Source: CAD feature listing. Evaluate the final solid. Frame: model axes, mm. A direction names the side the tool comes from. Round coordinates to 2 decimals unless told otherwise and drop trailing zeros. Write each loop counter-clockwise with the first axis right and the second up, starting at its lowest first coordinate (ties: lowest second). Pieces come first, ordered by that corner, then holes. Notation, with made-up numbers: M 47.5,-22.5 L 100.5,-22.5 A31 ccw 100.5,6.5 Z; hole C 82.5,68 d9. An arc over 180 degrees is marked long. Use a Markdown table: item, result.
```python
from build123d import *

# Parameters (mm, degrees)
SKETCH1_R           = 12
SKETCH1_R_2         = 5.5
BOSS_EXTRUDE1_DEPTH = 3
SKETCH1_5_R         = 5.5
SKETCH1_5_R_2       = 3
BOSS_EXTRUDE3_DEPTH = 12
FILLET2_R           = 2
CUT_EXTRUDE1_START  = -5.5
SKETCH2_R           = 1.6
CUT_EXTRUDE1_DEPTH  = 11
SKETCH3_R           = 2.001151749
CUT_EXTRUDE2_DEPTH  = 4


with BuildPart() as part:
    # Sketch1 → Boss-Extrude1 (new body)
    with BuildSketch(Plane.XY):
        Circle(SKETCH1_R)
        Circle(SKETCH1_R_2, mode=Mode.SUBTRACT)
    extrude(amount=BOSS_EXTRUDE1_DEPTH)

    # Sketch1<5> → Boss-Extrude3 (add)
    with BuildSketch(Plane.XY):
        Circle(SKETCH1_5_R)
        Circle(SKETCH1_5_R_2, mode=Mode.SUBTRACT)
    extrude(amount=BOSS_EXTRUDE3_DEPTH)

    # Fillet2
    fillet2_edges = [part.edges().sort_by_distance(p)[0] for p in [
        (-5.5, 0, 3),
    ]]
    fillet(fillet2_edges, radius=FILLET2_R)

    # Sketch2 → Cut-Extrude1 (cut)
    with BuildSketch(Plane(origin=(0, 0, 0), x_dir=(1, 0, 0), z_dir=(0, 1, 0)).offset(CUT_EXTRUDE1_START)):
        with Locations(Location((0, -7.949486667, 0), (0, 0, 90))):
            Circle(SKETCH2_R)
    extrude(amount=CUT_EXTRUDE1_DEPTH, mode=Mode.SUBTRACT)

    # Sketch3 → Cut-Extrude2 (cut)
    with BuildSketch(Plane.XY.offset(3)):
        with Locations((0, 8.599839423)):
            Circle(SKETCH3_R)
        with Locations((7.447679409, -4.299919712)):
            Circle(SKETCH3_R)
        with Locations((-7.447679409, -4.299919712)):
            Circle(SKETCH3_R)
    extrude(amount=-CUT_EXTRUDE2_DEPTH, mode=Mode.SUBTRACT)


solid = part.part
```
Q1. Reachability of faces 1 (the cylindrical face through (-8.923, -2.947, 1.521)), 2 (the cylindrical face through (5.08, -2.11, 8.45)), 3 (the flat face through (2.4, -2.4, 12)) from +Z, -Z, +X, -X, +Y, -Y: full face, straight path, thin tool, end or side. Return the list, or none.
Results are:
| item | result |
|---|---|
| face 1 | -Z |
| face 2 | +Z |
| face 3 | +Z, +X, -X, +Y, -Y |
Q2. Line query: L1, parallel to Y at x = 0, z = 0.7; L2, parallel to Z at x = 7.75, y = 7; L3, parallel to X at y = 3, z = 6.5. Output: solid intervals per line, ascending.
Results are:
| item | result |
|---|---|
| L1 | -12 to -3, 3 to 6.6, 10.6 to 12 |
| L2 | 0 to 3 |
| L3 | -4.61 to -0.68, 0.68 to 4.61 |
Q3. First-contact query: pin 1 Ø3 at (x, z) = (-6, 1) entering from +Y; pin 2 Ø2.5 at (x, y) = (-7.45, -4.3) entering from -Z; pin 3 Ø3.5 at (x, z) = (0, 7.95) entering from +Y. Flat tips, straight axial feed; report the tip coordinate or a pass-through.
Results are:
| item | result |
|---|---|
| pin 1 | y = 11.12 |
| pin 2 | z = 3 |
| pin 3 | y = 5.5 |
Q4. Section B-B on x = 0. Return loops of the section in (y, z).
Results are:
| item | result |
|---|---|
| outline | M -12,0 L -3,0 L -3,6.35 L -5.5,6.35 L -5.5,5 A2 cw -7.5,3 L -12,3 Z; M -5.5,9.55 L -3,9.55 L -3,12 L -5.5,12 Z; M 3,0 L 6.6,0 L 6.6,3 L 7.5,3 A2 cw 5.5,5 L 5.5,6.35 L 3,6.35 Z; M 3,9.55 L 5.5,9.55 L 5.5,12 L 3,12 Z; M 10.6,0 L 12,0 L 12,3 L 10.6,3 Z |
Q5. Section A-A on y = 0. Return loops of the section in (x, z), plus the area to 3 significant figures.
Results are:
| item | result |
|---|---|
| outline | M -12,0 L -3,0 L -3,12 L -5.5,12 L -5.5,5 A2 cw -7.5,3 L -12,3 Z; M 3,0 L 12,0 L 12,3 L 7.5,3 A2 cw 5.5,5 L 5.5,12 L 3,12 Z |
| area | 101 mm^2 |
Q6. Section C-C on z = 1. Return loops of the section in (x, y).
Results are:
| item | result |
|---|---|
| outline | C 0,0 d24; hole C -7.45,-4.3 d4; hole C 0,0 d6; hole C 0,8.6 d4; hole C 7.45,-4.3 d4 |
Q7. Mould query, pull axis Y, two halves, no side actions, for faces 4 (the flat face through (5, 6, 3)), 5 (the cylindrical face through (-11.99, 0.53, 1.48)), 6 (the cylindrical face through (7.187, -2.316, 1.521)). Classes: +Y half, -Y half, draft (parallel to the pull), parting line (faces both ways), or undercut.
Results are:
| item | result |
|---|---|
| face 4 | draft |
| face 5 | parting line |
| face 6 | undercut |
Q8. Section D-D on x = 9. Return loops of the section in (y, z), plus the area to 3 significant figures.
Results are:
| item | result |
|---|---|
| outline | M -7.94,0 L -5.56,0 L -5.56,3 L -7.94,3 Z; M -3.04,0 L 7.94,0 L 7.94,3 L -3.04,3 Z |
| area | 40.0 mm^2 |
